Geometry check sheet. Reference: drawing and pictorial views, mm from the part's lowest x, y, z. A direction names the side the tool comes from. Give positions to 0.01 mm unless a question says otherwise; leave off trailing zeros. Order: outer loops, then holes, each group sorted by start corner. A loop starts at its lowest first (then second) coordinate and runs counter-clockwise, first axis right, second up.
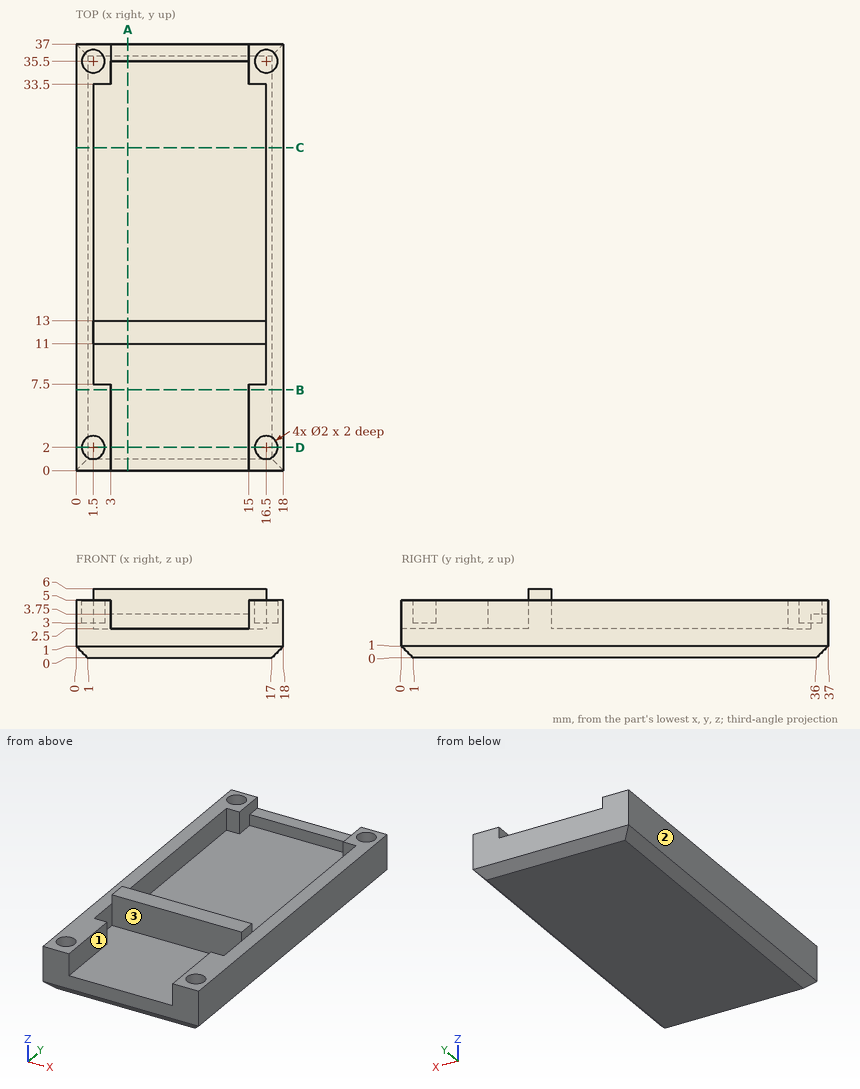
(1) Sectioned sample at B-B (y = 7). Enter the section's corners in (x, z), plus the area to 3 significant figures.
(2) Tool access check on the marked faces 1, 2 and 3. Record the directions out of +Z, -Z, +X, -X, +Y, -Y that give a thin tool (end or side, any length) a straight path to the whole face; none if there is none.
(3) Go/stop test with flat-tipped pins: P1, Ø1.6, axis at x = 1.5, y = 35.5, coming from the +Z side; P2, Ø5, axis at x = 15.5, y = 7, coming from the +Z side; P3, Ø1.8, axis at x = 10, z = 3.5, coming from the -Y side. Record where each tip stops, or that it passes through.
(4) Thickness scan on L1, parallel to Y at x = 2.75, z = 3.75; L2, parallel to X at y = 34, z = 3.5; L3, parallel to Z at x = 8.25, y = 4. Record the ranges inside material, lowest first.
(5) Sectioned sample at A-A (x = 4.5). Enter the section's corners in (y, z).
(6) Sectioned sample at C-C (y = 28). Enter the section's corners in (x, z).
(7) Sectioned sample at D-D (y = 2). Enter the section's corners in (x, z).
Values follow:
1. outline: (0, 1) - (1, 0) - (17, 0) - (18, 1) - (18, 5) - (15, 5) - (15, 2.5) - (3, 2.5) - (3, 5) - (0, 5) - close
1. area: 59.0 mm2
2. face 1: +Z, -Y
2. face 2: +Z, -Z, -X, +Y, -Y
2. face 3: +Z
3. P1: stops at z = 3
3. P2: stops at z = 5
3. P3: stops at y = 11
4. L1: y = 0 to 7.5, 11 to 13, 33.5 to 37
4. L2: x = 0 to 3, 15 to 18
4. L3: z = 0 to 2.5
5. outline: (0, 1) - (1, 0) - (36, 0) - (37, 1) - (37, 3.75) - (35.5, 3.75) - (35.5, 2.5) - (13, 2.5) - (13, 6) - (11, 6) - (11, 2.5) - (0, 2.5) - close
6. outline: (0, 1) - (1, 0) - (17, 0) - (18, 1) - (18, 5) - (16.5, 5) - (16.5, 2.5) - (1.5, 2.5) - (1.5, 5) - (0, 5) - close
7. outline: (0, 1) - (1, 0) - (17, 0) - (18, 1) - (18, 5) - (17.5, 5) - (17.5, 3) - (15.5, 3) - (15.5, 5) - (15, 5) - (15, 2.5) - (3, 2.5) - (3, 5) - (2.5, 5) - (2.5, 3) - (0.5, 3) - (0.5, 5) - (0, 5) - close
